```python
from build123d import *

# Parameters (mm, degrees)
SKETCH1_R                = 4.1
SKETCH1_R_2              = 4
SKETCH1_R_3              = 2.6
BOSS_EXTRUDE1_DEPTH      = 10
CUT_EXTRUDE1_START       = -4
CUT_EXTRUDE1_DEPTH       = 4
CUT_EXTRUDE2_REACH       = 113.917
BOSS_EXTRUDE2_DEPTH      = 10
BOSS_EXTRUDE2_DEPTH_BACK = 10
SKETCH5_R                = 4
FILLET1_R                = 1


with BuildPart() as part:
    # Sketch1 → Boss-Extrude1 (new body)
    with BuildSketch(Plane(origin=(0, 0, 0), x_dir=(1, 0, 0), z_dir=(0, 1, 0))):
        with BuildLine():
            Line((28.853428594, 9.206712552), (1.853428594, 9.206712552))
            ThreePointArc((1.853428594, 9.206712552), (-1.682105312, 10.671178646), (-3.146571406, 14.206712552))
            Line((-3.146571406, 14.206712552), (-3.146571406, 16.206712552))
            ThreePointArc((-3.146571406, 16.206712552), (-5.489717157, 21.863566801), (-11.146571406, 24.206712552))
            Line((-11.146571406, 24.206712552), (-15.146571406, 24.206712552))
            ThreePointArc((-15.146571406, 24.206712552), (-20.803425656, 21.863566801), (-23.146571406, 16.206712552))
            Line((-23.146571406, 16.206712552), (-23.146571406, -92.793287448))
            ThreePointArc((-23.146571406, -92.793287448), (-24.025251062, -94.914607792), (-26.146571406, -95.793287448))
            Line((-26.146571406, -95.793287448), (-40.146571406, -95.793287448))
            ThreePointArc((-40.146571406, -95.793287448), (-42.26789175, -94.914607792), (-43.146571406, -92.793287448))
            Line((-43.146571406, -92.793287448), (-43.146571406, 4.206712552))
            Line((-43.146571406, 4.206712552), (-43.146571406, 36.206712552))
            ThreePointArc((-43.146571406, 36.206712552), (-40.803425656, 41.863566801), (-35.146571406, 44.206712552))
            Line((-35.146571406, 44.206712552), (-3.146571406, 44.206712552))
            Line((-3.146571406, 44.206712552), (25.853428594, 44.206712552))
            ThreePointArc((25.853428594, 44.206712552), (31.510282843, 41.863566801), (33.853428594, 36.206712552))
            Line((33.853428594, 36.206712552), (33.853428594, 14.206712552))
            ThreePointArc((33.853428594, 14.206712552), (32.3889625, 10.671178646), (28.853428594, 9.206712552))
        make_face()
        with Locations(Location((25.853428594, 17.206712552, 0), (0, 0, 270))):
            Circle(SKETCH1_R, mode=Mode.SUBTRACT)
        with Locations(Location((4.853428594, 17.206712552, 0), (0, 0, 270))):
            Circle(SKETCH1_R_2, mode=Mode.SUBTRACT)
        with Locations(Location((-31.146571406, -87.793287448, 0), (0, 0, 270))):
            Circle(SKETCH1_R_3, mode=Mode.SUBTRACT)
        with Locations(Location((-31.146571406, -60.793287448, 0), (0, 0, 270))):
            Circle(SKETCH1_R_3, mode=Mode.SUBTRACT)
    extrude(amount=BOSS_EXTRUDE1_DEPTH)

    # Sketch2 → Cut-Extrude1 (cut)
    with BuildSketch(Plane(origin=(0, 10, 0), x_dir=(1, 0, 0), z_dir=(0, 1, 0)).offset(CUT_EXTRUDE1_START)):
        with BuildLine():
            Line((25.853428594, 24.706712552), (33.853428594, 24.706712552))
            Line((33.853428594, 24.706712552), (33.853428594, 14.206712552))
            ThreePointArc((33.853428594, 14.206712552), (32.3889625, 10.671178646), (28.853428594, 9.206712552))
            Line((28.853428594, 9.206712552), (18.353428594, 9.206712552))
            Line((18.353428594, 9.206712552), (18.353428594, 17.206712552))
            ThreePointArc((18.353428594, 17.206712552), (20.550127735, 22.510013411), (25.853428594, 24.706712552))
        make_face()
    extrude(amount=CUT_EXTRUDE1_DEPTH, mode=Mode.SUBTRACT)

    # Cut-Extrude2: up to this face of the body (flat: up to its plane)
    cut_extrude2_end = Plane(part.part.faces().sort_by_distance((-43.146571406, 5, 28.293287448))[0])
    # Sketch3 → Cut-Extrude2 (cut, up to the picked face)
    with BuildSketch(Plane(origin=(-23.146571406, 0, 0), x_dir=(0, 0, -1), z_dir=(1, 0, 0)), mode=Mode.PRIVATE) as cut_extrude2_sk1:
        Polygon((16.206712552, 10), (-48.793287448, 5), (-99.981688139, 5), (-99.981688139, 10), align=None)
    cut_extrude2_tool1 = split(extrude(cut_extrude2_sk1.sketch, amount=-CUT_EXTRUDE2_REACH, mode=Mode.PRIVATE), bisect_by=cut_extrude2_end, keep=Keep.BOTH, mode=Mode.PRIVATE)
    add(cut_extrude2_tool1.solids().sort_by(Axis((-23.146571, 7.823621, 56.033951), (-1, 0, 0)))[0], mode=Mode.SUBTRACT)

    # Sketch5 → Boss-Extrude2 (add, two sides: drawn at the far end of the back side and taken through both)
    with BuildSketch(Plane(origin=(0, 0, 0), x_dir=(-1, 0, 0), z_dir=(0, -1, 0)).offset(-BOSS_EXTRUDE2_DEPTH_BACK)):
        with Locations(Location((-4.853428594, 17.206712552, 0), (0, 0, 90))):
            Circle(SKETCH5_R)
    extrude(amount=BOSS_EXTRUDE2_DEPTH + BOSS_EXTRUDE2_DEPTH_BACK)

    # Fillet1
    fillet1_edges = [part.edges().sort_by_distance(p)[0] for p in [
        (4.853428594, 0, -13.206712552),
        (4.853428594, -10, -13.206712552),
    ]]
    fillet(fillet1_edges, radius=FILLET1_R)


solid = part.part
```
Input: part model. Units: mm. Frame: model coordinates. A direction names the side the tool comes from. Give positions to 0.01 mm unless a question says otherwise; leave off trailing zeros. Order: outer loops, then holes, each group sorted by start corner. A loop starts at its lowest first (then second) coordinate and runs counter-clockwise, first axis right, second up. Notation, with made-up numbers: (33.5, 12) -> (56.5, 12) arc R10 cw to (56.5, 27) -> close; hole circle Ø10 at (3, 77). An arc over 180 degrees is marked (long way). Write each question's results on one line, items separated by ' | '. Start each with the question number.
Item 1: Cut plane A-A on y = 2.5. Return the cut outline in (x, z), then the cut area to 3 significant figures.
Item 2: Cut plane B-B on z = 67. Return the cut outline in (x, y), then the cut area to 3 significant figures.
Item 3: Cut plane D-D on y = -6. Return the cut outline in (x, z), then the cut area to 3 significant figures.
Item 4: Mould query, pull axis X, two halves, no side actions, for faces 1 (the flat face through (30, 8, -24.707)), 2 (the flat face through (33.853, 4, -28)), 3 (the cylindrical face through (-33.453, 2.465, 88.993)). Classes: pulls with the +X half, pulls with the -X half, needs draft (parallel to the pull), parting line crosses it, or undercut.
Item 5: Contact query for flat-ended pins moving along their axis: P1, Ø7.5, axis at x = 28, z = -19, coming from the +Y side; P2, Ø2, axis at x = 30.5, y = 7.5, coming from the +Z side; P3, Ø11, axis at y = 4, z = 62.5, coming from the +X side. Output: stop coordinate, or through.
Item 6: Cut plane C-C on x = -1.5. Return the cut outline in (y, z).
Item 7: Set-up query: faces 4 (the flat face through (13, 4, -9.207)), 5 (the flat face through (-33, 5, 72)), 6 (the flat face through (-23.147, 4, 25)). Return all of +Z, -Z, +X, -X, +Y, -Y with unobstructed straight access to the full face (end or side cutting, diameter ignored); none if empty.
Item 8: Line query: line 1 (X direction, y = 7.25, z = -14); line 2 (Y direction, x = 23.5, z = -23); line 3 (Z direction, x = 14.5, y = 4). Output: solid intervals per line, ascending.
Established:
1) outline: (-43.15, -36.21) arc R8 ccw to (-35.15, -44.21) -> (25.85, -44.21) arc R8 ccw to (33.85, -36.21) -> (33.85, -14.21) arc R5 ccw to (28.85, -9.21) -> (1.85, -9.21) arc R5 ccw to (-3.15, -14.21) -> (-3.15, -16.21) arc R8 cw to (-11.15, -24.21) -> (-15.15, -24.21) arc R8 cw to (-23.15, -16.21) -> (-23.15, 92.79) arc R3 ccw to (-26.15, 95.79) -> (-40.15, 95.79) arc R3 ccw to (-43.15, 92.79) -> close; hole circle Ø5.2 at (-31.15, 60.79); hole circle Ø5.2 at (-31.15, 87.79); hole circle Ø8.2 at (25.85, -17.21) | area: 4,390 mm^2
2) outline: (-43.15, 0) -> (-23.15, 0) -> (-23.15, 5) -> (-43.15, 5) -> close | area: 100 mm^2
3) outline: circle Ø8 at (4.85, -17.21) | area: 50.3 mm^2
4) face 1: needs draft | face 2: pulls with the +X half | face 3: undercut
5) P1: y = 6 | P2: z = -24.71 | P3: x = -23.15
6) outline: (0, -44.21) -> (10, -44.21) -> (10, -10.5) -> (0, -10.5) -> close
7) face 4: +Z, +X, +Y, -Y | face 5: +Z, +X, -X, +Y | face 6: +Z, +Y, -Y
8) line 1: -43.15 to -23.15, -3.14 to 18.35 | line 2: 0 to 6 | line 3: -44.21 to -9.21
